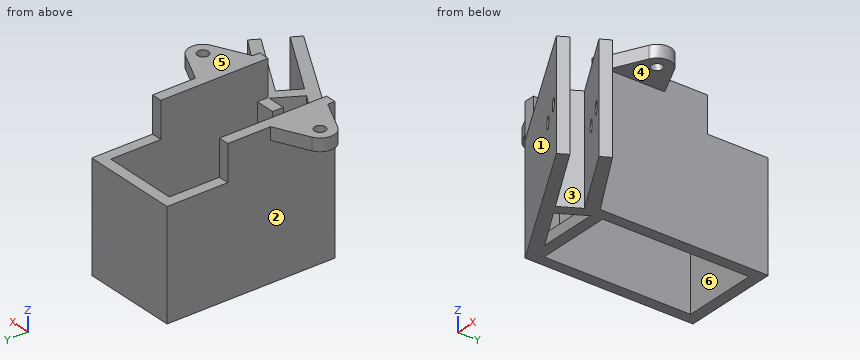
```python
from build123d import *

# Parameters (mm, degrees)
SKETCH_W        = 21
SKETCH_H        = 41
PAD_DEPTH       = 30
SKETCH001_W     = 10
SKETCH001_H     = 27
POCKET_DEPTH    = 3.1
SKETCH002_R     = 1.6
POCKET001_DEPTH = 12.5
SKETCH003_W     = 3
SKETCH003_H     = 30
PAD001_DEPTH    = 10
SKETCH004_R     = 1.55
PAD002_DEPTH    = 3.5


with BuildPart() as part:
    # Sketch → Pad (new body)
    with BuildSketch(Plane.XY):
        Polygon((13.5, 0), (13.5, 47), (-13.5, 47), (-13.5, 0), (26.918584287, -22.7583302492), (28.418584287, -20.1602540378), (8.5, -8.6602540378), (11.75, -3.0310889132), (31.668584287, -14.5310889132), (33.168584287, -11.9330127019), align=None)
        with Locations((0, 23.5)):
            Rectangle(SKETCH_W, SKETCH_H, mode=Mode.SUBTRACT)
        Polygon((-6.5, 0), (10.0358983849, 0), (5.9019237886, -7.1602540378), align=None, mode=Mode.SUBTRACT)
    extrude(amount=PAD_DEPTH)

    # Sketch001 (on Face11 of Pad) → Pocket (cut)
    with BuildSketch(Plane(origin=(0, 3, 0), x_dir=(-1, 0, 0), z_dir=(0, 1, 0))):
        with Locations((0, 16.5)):
            Rectangle(SKETCH001_W, SKETCH001_H)
    extrude(amount=-POCKET_DEPTH, mode=Mode.SUBTRACT)

    # Sketch002 (on Face10 of Pocket) → Pocket001 (cut, symmetric)
    with BuildSketch(Plane(origin=(-1.625, -2.8145825623, 0), x_dir=(-0.8660254038, 0.5, 0), z_dir=(0.5, 0.8660254038, 0))):
        with Locations((-30.1913429511, 15)):
            Circle(SKETCH002_R)
        with Locations((-22.1913429511, 15)):
            Circle(SKETCH002_R)
    extrude(amount=POCKET001_DEPTH, both=True, mode=Mode.SUBTRACT)

    # Sketch003 (on Face5 of Pocket001) → Pad001 (join)
    with BuildSketch(Plane.XY.offset(30)):
        with Locations((-12, 15)):
            Rectangle(SKETCH003_W, SKETCH003_H)
        with Locations((12, 15)):
            Rectangle(SKETCH003_W, SKETCH003_H)
    extrude(amount=PAD001_DEPTH)

    # Sketch004 (on Face26 of Pad001) → Pad002 (join)
    with BuildSketch(Plane.XY.offset(40)):
        with BuildLine():
            Line((-13.5, 18), (-13.5, 2))
            Line((-13.5, 2), (-22.7191621265, 6.3882855064))
            ThreePointArc((-22.7191621265, 13.6117144936), (-25, 10), (-22.7191621265, 6.3882855064))
            Line((-13.5, 18), (-22.7191621265, 13.6117144936))
        make_face()
        with Locations((-21, 10)):
            Circle(SKETCH004_R, mode=Mode.SUBTRACT)
        with BuildLine():
            Line((22.7191621265, 6.3882855064), (13.5, 2))
            Line((13.5, 2), (13.5, 18))
            Line((13.5, 18), (22.7191621265, 13.6117144936))
            ThreePointArc((22.7191621265, 6.3882855064), (25, 10), (22.7191621265, 13.6117144936))
        make_face()
        with Locations((21, 10)):
            Circle(SKETCH004_R, mode=Mode.SUBTRACT)
    extrude(amount=-PAD002_DEPTH)


solid = part.part
```
Verification items for the finished model (mm, model axes). Face numbers are marked on the shaded views. A direction names the side the tool comes from. Coordinates: 2 decimals unless noted, no trailing zeros. Write each loop counter-clockwise with the first axis right and the second up, starting at its lowest first coordinate (ties: lowest second). Pieces come first, ordered by that corner, then holes. Notation, with made-up numbers: (69, 22.25) - (95, 22.25) arc R28 cw to (95, 57.25) - close; hole circle Ø10 at (-9, -23). An arc over 180 degrees is marked (long way). One line per question, with ' | ' between items. Start each with the question number.
1. Material ranges on line 1 along X through (y, z) = (21, 37); line 2 along Y through (x, z) = (-21, 37); line 3 along Y through (x, z) = (4.5, 13), recorded low to high.
2. Section check A-A (y = 10). Enter the section's corners in (x, z).
3. Draft check along Y on the marked faces 1, 2 and 3. Enter one of: released by +Y, released by -Y, zero draft, split by the parting line, or undercut.
4. Gauge pin test, flat ends, axial feed: P1, Ø10, axis at y = 23.5, z = 11.5, coming from the -X side; P2, Ø3.5, axis at x = -12, z = 35, coming from the -Y side; P3, Ø5, axis at y = 13.5, z = 17, coming from the +X side; P4, Ø2, axis at x = -12.5, y = -4, coming from the +Z side. Record the tip position at first contact, or that the pin passes through.
5. Section check D-D (x = -21). Enter the section's corners in (y, z).
6. Section check C-C (y = 27). Enter the section's corners in (x, z).
7. Access from +Z, -Z, +X, -X, +Y, -Y to the whole of each face (thin tool, end or side, straight path). Record for the marked faces 4, 5 and 6.
8. Section check B-B (z = 20). Enter the section's corners in (x, y), plus the area to 3 significant figures.
Computed values:
1) line 1: -13.5 to -10.5, 10.5 to 13.5 | line 2: 5.57 to 8.45, 11.55 to 14.43 | line 3: -10.14 to -6.35, 44 to 47
2) outline: (-25, 36.5) - (-22.55, 36.5) - (-22.55, 40) - (-25, 40) - close; (-19.45, 36.5) - (-13.5, 36.5) - (-13.5, 0) - (-10.5, 0) - (-10.5, 40) - (-19.45, 40) - close; (10.5, 0) - (13.5, 0) - (13.5, 36.5) - (19.45, 36.5) - (19.45, 40) - (10.5, 40) - close; (22.55, 36.5) - (25, 36.5) - (25, 40) - (22.55, 40) - close
3) face 1: released by -Y | face 2: zero draft | face 3: undercut
4) P1: x = -13.5 | P2: y = 0 | P3: x = 13.5 | P4: through
5) outline: (5.57, 36.5) - (8.45, 36.5) - (8.45, 40) - (5.57, 40) - close; (11.55, 36.5) - (14.43, 36.5) - (14.43, 40) - (11.55, 40) - close
6) outline: (-13.5, 0) - (-10.5, 0) - (-10.5, 40) - (-13.5, 40) - close; (10.5, 0) - (13.5, 0) - (13.5, 40) - (10.5, 40) - close
7) face 4: -Z, +X, +Y, -Y | face 5: +Z, +X, -X, +Y, -Y | face 6: +Z, -Z
8) outline: (-13.5, 0) - (26.92, -22.76) - (28.42, -20.16) - (8.5, -8.66) - (11.75, -3.03) - (31.67, -14.53) - (33.17, -11.93) - (13.5, 0) - (13.5, 47) - (-13.5, 47) - close; hole (-10.5, 3) - (-5, 3) - (-5, 0) - (-6.5, 0) - (5.9, -7.16) - (10.04, 0) - (5, 0) - (5, 3) - (10.5, 3) - (10.5, 44) - (-10.5, 44) - close | area: 620 mm²
